Can you work these out from the model? Positions are in its coordinate system, mm. Face numbers are marked on the shaded views. Give positions to 0.01 mm unless a question says otherwise; leave off trailing zeros. Order: outer loops, then holes, each group sorted by start corner. A loop starts at its lowest first (then second) coordinate and runs counter-clockwise, first axis right, second up. Notation, with made-up numbers: (-17.75, 32.5) - (15.25, 32.5) arc R19 ccw to (15.25, 65.5) - close; hole circle Ø11 at (1, -37.5). An arc over 180 degrees is marked (long way). Use one line per item in the form item = value. Start each with the question number.
1) Please list where these lines run through material, in increasing order: probe 1 along Y at (x, z) = (-2.8, 0); probe 2 along Y at (x, z) = (-0.75, 6.25).
2) For pin 1 (1.5 mm diameter, centred on x = 1.5, z = 6, fed in from -Y); pin 2 (1 mm diameter, centred on x = -2.5, z = -2.5, fed in from +Y); pin 3 (4 mm diameter, centred on x = 0, y = 5, fed in from -Z), each with a flat end and sliding along its axis, tell me the tip position at first contact or that it passes through.
3) We'd pull the mould along Z, two halves only. Please class the marked faces 1, 2 and 3: released by +Z, released by -Z, zero draft, split by the parting line, or undercut.
4) Suppose I cut it at A-A, the plane y = 0. Write out the boundary of the cut face in (x, z), and give its area (3 significant figures).
```python
from build123d import *

# Parameters (mm, degrees)
FILLET1_R = 0.5


with BuildPart() as part:
    # Sketch2 → Revolve1 (revolve)
    with BuildSketch(Plane.XY):
        with BuildLine():
            Line((3.5, 9.6), (3.5, 11))
            Line((3.5, 11), (-3.5, 11))
            Line((-3.5, 11), (-3.5, 9.6))
            Line((-3.5, 9.6), (-0.835607713, 9.6))
            ThreePointArc((-0.835607713, 9.6), (0, 9.7845), (0.835607713, 9.6))
            Line((0.835607713, 9.6), (3.5, 9.6))
        make_face()
    revolve(axis=Axis((23.660185957, 0, 0), (-1, 0, 0)))

    # Fillet1
    fillet1_edges = [part.edges().sort_by_distance(p)[0] for p in [
        (-3.5, -11, 0),
        (3.5, -11, 0),
    ]]
    fillet(fillet1_edges, radius=FILLET1_R)


solid = part.part
```
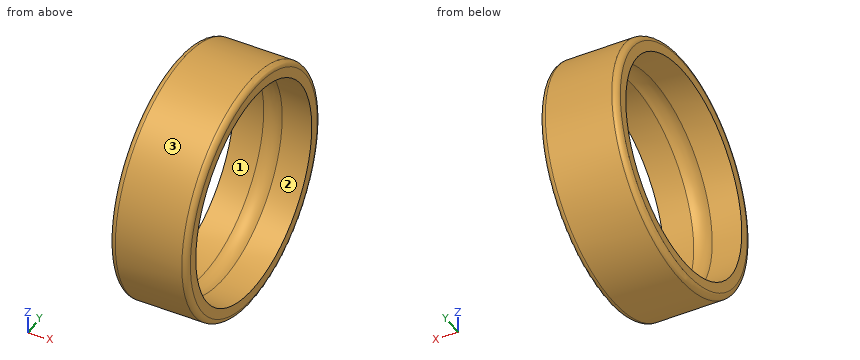
Result sheet:
q1.probe_1 = -11 to -9.6, 9.6 to 11
q1.probe_2 = -9.05 to -7.34, 7.34 to 9.05
q2.pin_1 = -9.67
q2.pin_2 = 10.82
q2.pin_3 = -10.58
q3.face_1 = undercut
q3.face_2 = undercut
q3.face_3 = split by the parting line
q4.outline = (-3.5, -10.5) arc R0.5 ccw to (-3, -11) - (3, -11) arc R0.5 ccw to (3.5, -10.5) - (3.5, -9.6) - (0.84, -9.6) arc R1.98 cw to (-0.84, -9.6) - (-3.5, -9.6) - close; (-3.5, 9.6) - (-0.84, 9.6) arc R1.98 cw to (0.84, 9.6) - (3.5, 9.6) - (3.5, 10.5) arc R0.5 ccw to (3, 11) - (-3, 11) arc R0.5 ccw to (-3.5, 10.5) - close
q4.area = 19.0 mm²
